```python
from build123d import *

# Parameters (mm, degrees)
BOSS_EXTRUDE1_DEPTH = 45
SKETCH3_R           = 130
CUT_EXTRUDE1_DEPTH  = 1019.38418632
SKETCH2_R           = 130
CUT_EXTRUDE2_DEPTH  = 1019.38418632


with BuildPart() as part:
    # Sketch1 → Boss-Extrude1 (new, symmetric)
    with BuildSketch(Plane.XY):
        with BuildLine():
            ThreePointArc((-433.012701892, 0), (-649.519052838, -375), (-216.506350946, -375))
            ThreePointArc((-216.506350946, -375), (0, -250), (216.506350946, -375))
            ThreePointArc((216.506350946, -375), (649.519052838, -375), (433.012701892, 0))
            ThreePointArc((433.012701892, 0), (216.506350946, 125), (216.506350946, 375))
            ThreePointArc((216.506350946, 375), (0, 750), (-216.506350946, 375))
            ThreePointArc((-216.506350946, 375), (-216.506350946, 125), (-433.012701892, 0))
        make_face()
    extrude(amount=BOSS_EXTRUDE1_DEPTH, both=True)

    # Sketch3 → Cut-Extrude1 (cut, through all)
    with BuildSketch(Plane(origin=(0, 0, -45), x_dir=(-1, 0, 0), z_dir=(0, 0, -1))):
        Circle(SKETCH3_R)
    extrude(amount=-CUT_EXTRUDE1_DEPTH, mode=Mode.SUBTRACT)

    # Sketch2 → Cut-Extrude2 (cut, through all)
    with BuildSketch(Plane.XY.offset(45)):
        with Locations((-433.012701892, -250)):
            Circle(SKETCH2_R)
        with Locations((433.012701892, -250)):
            Circle(SKETCH2_R)
        with Locations((0, 500)):
            Circle(SKETCH2_R)
    extrude(amount=-CUT_EXTRUDE2_DEPTH, mode=Mode.SUBTRACT)


solid = part.part
```
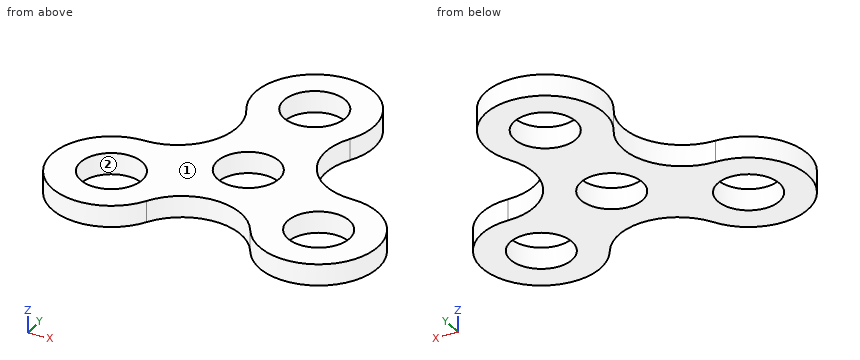
Part model, mm, in its own coordinate system. Face numbers are marked on the shaded views. Round coordinates to 2 decimals unless told otherwise and drop trailing zeros. Loops run counter-clockwise (first coordinate to the right, second up) from the corner with the lowest first, then second, coordinate; pieces in that order, holes last. Notation, with made-up numbers: (23, -2.75) -> (37, -2.75) arc R15 ccw to (37, 7.25) -> close; hole circle Ø10 at (7.25, 17.25). An arc over 180 degrees is marked (long way). Use one line per item in the form item = value. Start each with the question number.
Item 1: Band-saw the part on C-C (x = -351). List the corners of the cut face in (y, z).
Item 2: Band-saw the part on A-A (z = 15). List the corners of the cut face in (x, y), plus the area to 3 significant figures.
Item 3: Two-plate mould, pull along X, no slides. Class the marked faces 1 and 2: released by +X, released by -X, zero draft, split by the parting line, or undercut.
Item 4: Band-saw the part on B-B (y = 566). List the corners of the cut face in (x, z).
Item 5: Drill centre lines: line 1 along Y through (x, z) = (0, -13); line 2 along Y through (x, z) = (32, -29.5); line 3 along X through (y, z) = (-144, 21). Where is each one in solid material? Low to high.
Item 6: Drop flat-ended pins along their axis: pin 1 Ø5 at (y, z) = (-363, 17.5) entering from +X; pin 2 Ø5 at (x, z) = (-25, -11) entering from +Y; pin 3 Ø4 at (x, z) = (510, 13) entering from -Y. Give the stop position or say it passes through.
Item 7: Band-saw the part on D-D (y = 260). List the corners of the cut face in (x, z).
Data:
q1.outline = (-486.17, -45) -> (-350.87, -45) -> (-350.87, 45) -> (-486.17, 45) -> close; (-149.13, -45) -> (13.83, -45) -> (13.83, 45) -> (-149.13, 45) -> close
q2.outline = (-433.01, 0) arc R250 ccw (long way) to (-216.51, -375) arc R250 cw to (216.51, -375) arc R250 ccw (long way) to (433.01, 0) arc R250 cw to (216.51, 375) arc R250 ccw (long way) to (-216.51, 375) arc R250 cw to start; hole circle Ø260 at (-433.01, -250); hole circle Ø260 at (0, 0); hole circle Ø260 at (0, 500); hole circle Ø260 at (433.01, -250)
q2.area = 633,000 mm^2
q3.face_1 = zero draft
q3.face_2 = undercut
q4.outline = (-241.13, -45) -> (-112, -45) -> (-112, 45) -> (-241.13, 45) -> close; (112, -45) -> (241.13, -45) -> (241.13, 45) -> (112, 45) -> close
q5.line_1 = -250 to -130, 130 to 370, 630 to 750
q5.line_2 = -252.06 to -126, 126 to 374, 626 to 747.94
q5.line_3 = -659.43 to -508.27, -357.75 to 357.75, 508.27 to 659.43
q6.pin_1 = 657.27
q6.pin_2 = 748.99
q6.pin_3 = -488.49
q7.outline = (-183.21, -45) -> (183.21, -45) -> (183.21, 45) -> (-183.21, 45) -> close
